The model under review builds one solid part; all positions refer to its coordinate system, in mm. Give positions to 0.01 mm unless a question says otherwise; leave off trailing zeros. Write each loop counter-clockwise with the first axis right and the second up, starting at its lowest first coordinate (ties: lowest second). Pieces come first, ordered by that corner, then holes. Notation, with made-up numbers: (11, 21.25) -> (25, 21.25) arc R35 cw to (25, 55.25) -> close; hole circle Ø8 at (-5.5, 0). An arc over 180 degrees is marked (long way). Use CSV: the item, a comma, the result in double quotes.
```python
from build123d import *

# Parameters (mm, degrees)
SKETCH_R  = 80
SKETCH_W  = 5
SKETCH_H  = 12
PAD_DEPTH = 3


with BuildPart() as part:
    # Sketch → Pad (new body)
    with BuildSketch(Plane.XY):
        Circle(SKETCH_R)
        with Locations((-47.5, 0)):
            Rectangle(SKETCH_W, SKETCH_H, mode=Mode.SUBTRACT)
        with Locations((47.5, 0)):
            Rectangle(SKETCH_W, SKETCH_H, mode=Mode.SUBTRACT)
    extrude(amount=PAD_DEPTH)


solid = part.part
```
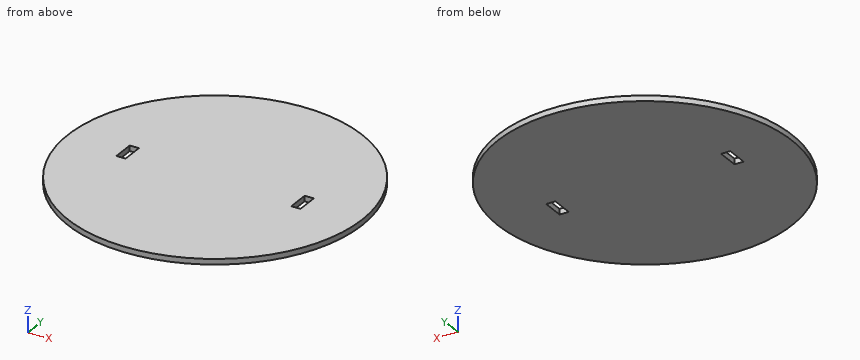
Q1. Consider section D-D (y = 18). Write out the cut boundary in (x, z), then the cut area to 3 significant figures.
Derived:
outline,"(-77.95, 0) -> (77.95, 0) -> (77.95, 3) -> (-77.95, 3) -> close"
area,"468 mm2"
Q2. Consider section C-C (x = 39). Write out the cut boundary in (y, z), then the cut area to 3 significant figures.
Derived:
outline,"(-69.85, 0) -> (69.85, 0) -> (69.85, 3) -> (-69.85, 3) -> close"
area,"419 mm2"
Q3. To check wall thickness, follow probe 1 along X at (y, z) = (3, 1.85); probe 2 along Y at (x, z) = (-2, 0.55) (3 decimals); probe 3 along Y at (x, z) = (-47.5, 2.2). State the ranges of each line that lie inside material, in increasing order.
Derived:
probe 1,"x = -79.94 to -50, -45 to 45, 50 to 79.94"
probe 2,"y = -79.975 to 79.975"
probe 3,"y = -64.37 to -6, 6 to 64.37"
Q4. Consider section A-A (y = 0). Write out the cut boundary in (x, z).
Derived:
outline,"(-80, 0) -> (-50, 0) -> (-50, 3) -> (-80, 3) -> close; (-45, 0) -> (45, 0) -> (45, 3) -> (-45, 3) -> close; (50, 0) -> (80, 0) -> (80, 3) -> (50, 3) -> close"
Q5. Insertion check: pin 1 (4 mm diameter, centred on x = 7.5, y = 32, fed in from -Z); pin 2 (1.5 mm diameter, centred on y = 3, z = 1.5, fed in from +X); pin 3 (1.5 mm diameter, centred on x = 47.5, z = 1, fed in from -Y). Each pin has a flat end and moves straight along its axis. Give the tip position at first contact, or say it passes through.
Derived:
pin 1,"stops at z = 0"
pin 2,"stops at x = 79.97"
pin 3,"stops at y = -64.92"
Q6. Consider section B-B (z = 0.95). Write out the cut boundary in (x, y).
Derived:
outline,"circle Ø160 at (0, 0); hole (-50, -6) -> (-45, -6) -> (-45, 6) -> (-50, 6) -> close; hole (45, -6) -> (50, -6) -> (50, 6) -> (45, 6) -> close"
